Part model, mm, in its own coordinate system. Give positions to 0.01 mm unless a question says otherwise; leave off trailing zeros. Write each loop counter-clockwise with the first axis right and the second up, starting at its lowest first coordinate (ties: lowest second). Pieces come first, ordered by that corner, then holes. Notation, with made-up numbers: M -2.75,77.5 L 17.25,77.5 A20 ccw 17.25,98.5 Z; hole C 41,-1 d3. An arc over 180 degrees is marked long. Use a Markdown table: item, result. Add a question column.
from build123d import *

# Parameters (mm, degrees)
SKETCH1_W                                = 369.57380619
SKETCH1_H                                = 64
BOSS_EXTRUDE1_DEPTH                      = 9.525
F_15_32_0_475_DIAMETER_HOLE1_D           = 12.065
F_15_32_0_475_DIAMETER_HOLE1_DEPTH       = 10.1092
F_15_32_0_475_DIAMETER_HOLE1_CSINK_D     = 13.17625
F_15_32_0_475_DIAMETER_HOLE1_CSINK_ANGLE = 100
F_15_32_0_475_DIAMETER_HOLE1_TIP         = 3.624691684
M4X0_7_TAPPED_HOLE1_D                    = 3.3
M4X0_7_TAPPED_HOLE1_CSINK_D              = 4.05
M4X0_7_TAPPED_HOLE1_CSINK_ANGLE          = 100


with BuildPart() as part:
    # Sketch1 → Boss-Extrude1 (new body)
    with BuildSketch(Plane(origin=(0, 0, 0), x_dir=(1, 0, 0), z_dir=(0, 1, 0))):
        with Locations((184.786903095, 32)):
            Rectangle(SKETCH1_W, SKETCH1_H)
    extrude(amount=BOSS_EXTRUDE1_DEPTH)

    # 15/32 (0.475) Diameter Hole1
    with Locations(Plane(origin=(0, 9.525, 0), x_dir=(1, 0, 0), z_dir=(0, 1, 0))):
        with Locations((350.52380619, 32)):
            CounterSinkHole(F_15_32_0_475_DIAMETER_HOLE1_D / 2, F_15_32_0_475_DIAMETER_HOLE1_CSINK_D / 2, depth=F_15_32_0_475_DIAMETER_HOLE1_DEPTH, counter_sink_angle=F_15_32_0_475_DIAMETER_HOLE1_CSINK_ANGLE)
            with Locations((0, 0, -(F_15_32_0_475_DIAMETER_HOLE1_DEPTH + F_15_32_0_475_DIAMETER_HOLE1_TIP / 2))):  # 118° drill point
                Cone(0, F_15_32_0_475_DIAMETER_HOLE1_D / 2, F_15_32_0_475_DIAMETER_HOLE1_TIP, mode=Mode.SUBTRACT)

    # M4x0.7 Tapped Hole1 (through all)
    with Locations(Plane(origin=(0, 9.525, 0), x_dir=(1, 0, 0), z_dir=(0, 1, 0))):
        with Locations((49, 44), (49, 20), (5, 44), (5, 20)):
            CounterSinkHole(M4X0_7_TAPPED_HOLE1_D / 2, M4X0_7_TAPPED_HOLE1_CSINK_D / 2, counter_sink_angle=M4X0_7_TAPPED_HOLE1_CSINK_ANGLE)

    # Sketch11 → CBORE for 1/4 Socket Head Cap Screw1 (revolve, cut)
    with BuildSketch(Plane(origin=(23.5, 9.525, -32), x_dir=(0, 0, 1), z_dir=(1, 0, 0))):
        Polygon((0, 0), (0, 9.525), (3.3782, 9.525), (3.3782, 6.35), (5.55625, 6.35), (5.55625, 0.532828266), (6.19125, 0), align=None)
    revolve(axis=Axis((23.5, 15.875, -32), (0, -1, 0)), mode=Mode.SUBTRACT)


solid = part.part
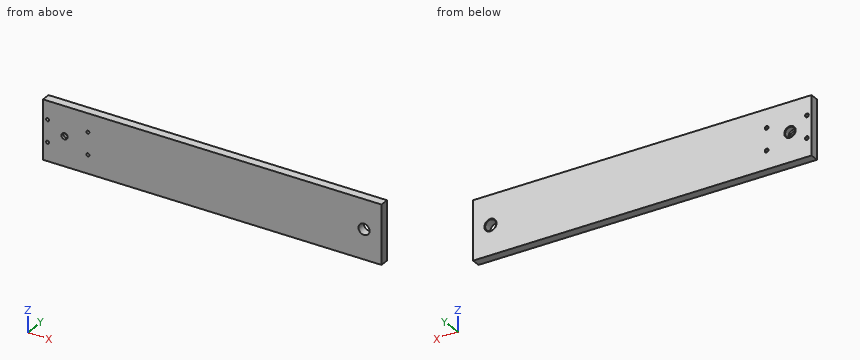
1. Cut at B-B (z = -32). Write the cut outline in (x, y) (3 decimals).
2. Drill centre lines: probe 1 along Z at (x, y) = (49, 3.25); probe 2 along X at (y, z) = (5.5, -32); probe 3 along X at (y, z) = (6.75, -43.5). Where is each one in solid material? Low to high. Write a range as [from, to].
3. Cut at A-A (x = 23.5). Write the cut outline in (y, z) (3 decimals), then the cut area to 3 significant figures.
4. Flat gauge pins, fed straight in: pin 1 (2.5 mm diameter, centred on x = 49, z = -20, fed in from -Y); pin 2 (10 mm diameter, centred on x = 23.5, z = -32, fed in from +Y) (3 decimals). Where does each tip first touch, or does it go through?
A:
| question | item | result |
|---|---|---|
| 1 | outline | M 0,0 L 20.122,0 L 20.122,3.175 L 17.944,3.175 L 17.944,8.992 L 17.309,9.525 L 0,9.525 Z; M 26.878,0 L 344.491,0 L 344.491,9.059 L 343.936,9.525 L 29.691,9.525 L 29.056,8.992 L 29.056,3.175 L 26.878,3.175 Z; M 356.556,0 L 369.574,0 L 369.574,9.525 L 357.112,9.525 L 356.556,9.059 Z |
| 2 | probe 1 | z = [-64, -45.65], [-42.35, -21.65], [-18.35, 0] |
| 2 | probe 2 | x = [0, 17.94], [29.06, 344.49], [356.56, 369.57] |
| 2 | probe 3 | x = [0, 3.43], [6.57, 47.43], [50.57, 369.57] |
| 3 | outline | M 0,-64 L 9.525,-64 L 9.525,-38.191 L 8.992,-37.556 L 3.175,-37.556 L 3.175,-35.378 L 0,-35.378 Z; M 0,-28.622 L 3.175,-28.622 L 3.175,-26.444 L 8.992,-26.444 L 9.525,-25.809 L 9.525,0 L 0,0 Z |
| 3 | area | 517 mm² |
| 4 | pin 1 | passes through |
| 4 | pin 2 | stops at y = 3.175 |
